from build123d import *

# Parameters (mm, degrees)
SKETCH2_W          = 39.2
SKETCH2_H          = 39.2
CUT_EXTRUDE1_DEPTH = 7


with BuildPart() as part:
    # Sketch1 → Revolve1 (revolve)
    with BuildSketch(Plane.XY, mode=Mode.PRIVATE) as revolve1_sk:
        with BuildLine():
            Line((-7, 0), (-7, 8.5))
            Line((-7, 8.5), (-6.24944465, 9.8))
            Line((-6.24944465, 9.8), (0, 9.8))
            Line((0, 9.8), (0, 5.5))
            ThreePointArc((0, 5.5), (0.146446609, 5.146446609), (0.5, 5))
            Line((0.5, 5), (49.3865, 5))
            Line((49.3865, 5), (50, 4.3865))
            Line((50, 4.3865), (50, 0))
            Line((50, 0), (-7, 0))
        make_face()
    revolve(revolve1_sk.sketch.rotate(Axis((50, 0, 0), (-1, 0, 0)), 270), axis=Axis((50, 0, 0), (-1, 0, 0)))

    # Sketch2 → Cut-Extrude1 (cut)
    with BuildSketch(Plane(origin=(0, 0, 0), x_dir=(0, 0, -1), z_dir=(1, 0, 0))):
        Rectangle(SKETCH2_W, SKETCH2_H)
        Polygon((-8.5, 4.907477288), (-8.5, -4.907477288), (0, -9.814954576), (8.5, -4.907477288), (8.5, 4.907477288), (0, 9.814954576), align=None, mode=Mode.SUBTRACT)
    extrude(amount=-CUT_EXTRUDE1_DEPTH, mode=Mode.SUBTRACT)


solid = part.part
Build history of the part. All positions in model axes, mm. A direction names the side the tool comes from. Round coordinates to 2 decimals unless told otherwise and drop trailing zeros. Write each loop counter-clockwise with the first axis right and the second up, starting at its lowest first coordinate (ties: lowest second). Pieces come first, ordered by that corner, then holes. Notation, with made-up numbers: (69.25, 15) -> (107.25, 15) arc R27 cw to (107.25, 40) -> close; hole circle Ø11 at (57, 62.5). An arc over 180 degrees is marked (long way). Use one line per item in the form item = value.
Q1. Band-saw the part on A-A, the plane x = 39.5. Write the cut outline in (y, z).
Conclusion:
outline = circle Ø10 at (0, 0)
Q2. Drop flat-ended pins along their axis: P1, Ø3, axis at x = 0.5, z = -6.5, coming from the -Y side; P2, Ø8, axis at x = 39.5, z = 3, coming from the +Y side; P3, Ø6, axis at y = 7.5, z = 6, coming from the +X side. Give the stop position or say it passes through.
Conclusion:
P1 = -6.88
P2 = 5
P3 = 0
Q3. Drill centre lines: L1, parallel to X at y = 1, z = -7.5; L2, parallel to X at y = -3.25, z = 3.5; L3, parallel to Z at x = 27, y = 0.75. Where is each one in solid material? Low to high.
Conclusion:
L1 = -7 to 0
L2 = -7 to 49.61
L3 = -4.94 to 4.94
Q4. Tool access for faces 1 (the conical face through (-6.79, -8.86, -0.02)), 2 (the cylindrical face through (25.29, -4.88, -1.08)): list every direction of +Z, -Z, +X, -X, +Y, -Y with a clear straight run to the whole face (end or side of a thin tool).
Conclusion:
face_1 = -X, -Y
face_2 = +X
